from build123d import *

# Parameters (mm, degrees)
F1_DEPTH      = 1409.446
F3_DEPTH      = 50.801
F3_DEPTH_BACK = 50.801
F4_R          = 6.35
F5_DEPTH      = 25.4


with BuildPart() as f1:
    # F0 (on Right) → F1 (new body)
    with BuildSketch(Plane.YZ):
        with BuildLine():
            Line((-47.625, -25.4), (47.625, -25.4))
            ThreePointArc((47.625, -25.4), (49.8700640303, -24.4700640303), (50.8, -22.225))
            Line((50.8, -22.225), (50.8, 22.225))
            ThreePointArc((50.8, 22.225), (49.8700640303, 24.4700640303), (47.625, 25.4))
            Line((47.625, 25.4), (-47.625, 25.4))
            ThreePointArc((-47.625, 25.4), (-49.8700640303, 24.4700640303), (-50.8, 22.225))
            Line((-50.8, 22.225), (-50.8, -22.225))
            ThreePointArc((-50.8, -22.225), (-49.8700640303, -24.4700640303), (-47.625, -25.4))
        make_face()
        with BuildLine():
            Line((-44.45, 22.225), (44.45, 22.225))
            ThreePointArc((44.45, 22.225), (46.6950640303, 21.2950640303), (47.625, 19.05))
            Line((47.625, 19.05), (47.625, -19.05))
            ThreePointArc((47.625, -19.05), (46.6950640303, -21.2950640303), (44.45, -22.225))
            Line((44.45, -22.225), (-44.45, -22.225))
            ThreePointArc((-44.45, -22.225), (-46.6950640303, -21.2950640303), (-47.625, -19.05))
            Line((-47.625, -19.05), (-47.625, 19.05))
            ThreePointArc((-47.625, 19.05), (-46.6950640303, 21.2950640303), (-44.45, 22.225))
        make_face(mode=Mode.SUBTRACT)
    extrude(amount=F1_DEPTH)

    # F2 (on Front) → F3 (cut, two sides)
    with BuildSketch(Plane.XZ) as f3_sk:
        Polygon((0, 25.4), (0, -25.4), (35.5705429411, -25.4), align=None)
        Polygon((1409.446, 25.4), (1373.8754570589, -25.4), (1409.446, -25.4), align=None)
    extrude(amount=-F3_DEPTH, mode=Mode.SUBTRACT)
    extrude(f3_sk.sketch, amount=F3_DEPTH_BACK, mode=Mode.SUBTRACT)

    # F4 (on face) → F5 (cut)
    with BuildSketch(Plane.XY.offset(25.4)):
        with Locations((19.05, 0)):
            Circle(F4_R)
        with Locations((1390.396, 0)):
            Circle(F4_R)
    extrude(amount=-F5_DEPTH, mode=Mode.SUBTRACT)


solid = f1.part
Read the model definition and answer for the solid it produces. Units are mm, in the model's axes. A direction names the side the tool comes from. Give positions to 0.01 mm unless a question says otherwise; leave off trailing zeros. Loops run counter-clockwise (first coordinate to the right, second up) from the corner with the lowest first, then second, coordinate; pieces in that order, holes last. Notation, with made-up numbers: (76, 65) -> (86, 65) arc R25 ccw to (86, 85) -> close; hole circle Ø11 at (83.25, 73). An arc over 180 degrees is marked (long way). Use a Markdown table: item, result.
Q1. A tool of negligible diameter and unlimited length cuts with its end or side. For faces 4 (the face through (695, 47.625, 0)), 5 (the face through (33.68, 4, -22.7)), from which of +Z, -Z, +X, -X, +Y, -Y can it reach the whole face along a straight path? Write none if from no direction.
Solved:
| item | result |
|---|---|
| face 4 | +X, -X |
| face 5 | -Z, -X, +Y, -Y |
Q2. Section B-B, the plane x = 859.5 is taken. Determine the outline of the cut face in (y, z) (3 decimals), then the cut area to 3 significant figures.
Solved:
| item | result |
|---|---|
| outline | (-50.8, -22.225) arc R3.175 ccw to (-47.625, -25.4) -> (47.625, -25.4) arc R3.175 ccw to (50.8, -22.225) -> (50.8, 22.225) arc R3.175 ccw to (47.625, 25.4) -> (-47.625, 25.4) arc R3.175 ccw to (-50.8, 22.225) -> close; hole (-47.625, -19.05) arc R3.175 ccw to (-44.45, -22.225) -> (44.45, -22.225) arc R3.175 ccw to (47.625, -19.05) -> (47.625, 19.05) arc R3.175 ccw to (44.45, 22.225) -> (-44.45, 22.225) arc R3.175 ccw to (-47.625, 19.05) -> close |
| area | 927 mm^2 |
Q3. Section A-A, the plane y = 27.5 is taken. Determine the outline of the cut face in (x, z) (3 decimals), then the cut area to 3 significant figures.
Solved:
| item | result |
|---|---|
| outline | (0, 25.4) -> (2.223, 22.225) -> (1407.223, 22.225) -> (1409.446, 25.4) -> close; (33.347, -22.225) -> (35.571, -25.4) -> (1373.875, -25.4) -> (1376.099, -22.225) -> close |
| area | 8,720 mm^2 |
Q4. Determine the mould class of faces 1 (the face through (695, 1, 25.4)), 2 (the face through (695, -1, 22.225)), 3 (the face through (695, -1, -25.4)) for opening direction Z: pulls with the +Z half, pulls with the -Z half, needs draft (parallel to the pull), parting line crosses it, or undercut.
Solved:
| item | result |
|---|---|
| face 1 | pulls with the +Z half |
| face 2 | undercut |
| face 3 | pulls with the -Z half |
Q5. Find the intervals of material crossed by line 1 along Y through (x, z) = (143, 5) (3 decimals); line 2 along Z through (x, y) = (589.5, -24.5) (3 decimals); line 3 along Y through (x, z) = (19, 23), in increasing order.
Solved:
| item | result |
|---|---|
| line 1 | y = -50.8 to -47.625, 47.625 to 50.8 |
| line 2 | z = -25.4 to -22.225, 22.225 to 25.4 |
| line 3 | y = -50.7 to -6.35, 6.35 to 50.7 |
Q6. Each of these flat-tipped pins is pushed along its axis until it touches: pin 1 (20.5 mm diameter, centred on x = 19.05, y = 0, fed in from -Z) (3 decimals); pin 2 (10 mm diameter, centred on y = -7.5, z = 18, fed in from -X). Where does it stop, or does it pass through?
Solved:
| item | result |
|---|---|
| pin 1 | stops at z = 22.225 |
| pin 2 | stops at x = 1.68 |
Q7. Section C-C, the plane z = -2 is taken. Determine the outline of the cut face in (x, y) (3 decimals), then the cut area to 3 significant figures.
Solved:
| item | result |
|---|---|
| outline | (19.186, -50.8) -> (1390.26, -50.8) -> (1390.26, -47.625) -> (19.186, -47.625) -> close; (19.186, 47.625) -> (1390.26, 47.625) -> (1390.26, 50.8) -> (19.186, 50.8) -> close |
| area | 8,710 mm^2 |
